Build history of the part. All positions in model axes, mm. Round coordinates to 2 decimals unless told otherwise and drop trailing zeros. Write each loop counter-clockwise with the first axis right and the second up, starting at its lowest first coordinate (ties: lowest second). Pieces come first, ordered by that corner, then holes.
Item 1: Band-saw the part on B-B, the plane z = 2.7. Count the separate pieces of the cut face and the enclosed holes in it, then the cut area to 3 significant figures.
Item 2: Drop flat-ended pins along their axis: pin 1 Ø12 at (x, y) = (-149.3, 205.49) entering from -Z; pin 2 Ø9.5 at (x, y) = (-149.3, -205.49) entering from -Z; pin 3 Ø2 at (x, z) = (-147.5, 2.5) entering from +Y; pin 4 Ø1.5 at (y, z) = (166, 3.5) entering from +X. Give the stop position or say it passes through.
Item 3: Band-saw the part on A-A, the plane y = 0. Write the cut outline in (x, z).
Item 4: Band-saw the part on C-C, the plane x = -118. Write the cut outline in (y, z), then the cut area to 3 significant figures.
Item 5: Wall check: probe 1 along Y at (x, z) = (0, 3.3); probe 2 along Y at (x, z) = (-146.5, 0.6); probe 3 along X at (y, z) = (-77, 5.5). Give the ranges that are in metal, low to high.
Item 6: Band-saw the part on D-D, the plane y = -107. Write the cut outline in (x, z).
```python
from build123d import *

# Parameters (mm, degrees)
F0_R     = 300
F0_R_2   = 5.25
F0_R_3   = 26
F1_DEPTH = 6


with BuildPart() as f1:
    # F0 (on Top) → F1 (new body)
    with BuildSketch(Plane.XY):
        Circle(F0_R)
        with Locations((-149.297454, -205.490317)):
            Circle(F0_R_2, mode=Mode.SUBTRACT)
        with Locations((-241.568355, -78.490317)):
            Circle(F0_R_2, mode=Mode.SUBTRACT)
        with Locations((0, -254)):
            Circle(F0_R_2, mode=Mode.SUBTRACT)
        with Locations((149.297454, -205.490317)):
            Circle(F0_R_2, mode=Mode.SUBTRACT)
        with Locations((241.568355, -78.490317)):
            Circle(F0_R_2, mode=Mode.SUBTRACT)
        with Locations((-241.568355, 78.490317)):
            Circle(F0_R_2, mode=Mode.SUBTRACT)
        with Locations((-149.297454, 205.490317)):
            Circle(F0_R_2, mode=Mode.SUBTRACT)
        Circle(F0_R_3, mode=Mode.SUBTRACT)
        with Locations((241.568355, 78.490317)):
            Circle(F0_R_2, mode=Mode.SUBTRACT)
        with Locations((149.297454, 205.490317)):
            Circle(F0_R_2, mode=Mode.SUBTRACT)
        with Locations((0, 254)):
            Circle(F0_R_2, mode=Mode.SUBTRACT)
    extrude(amount=F1_DEPTH)


solid = f1.part
```
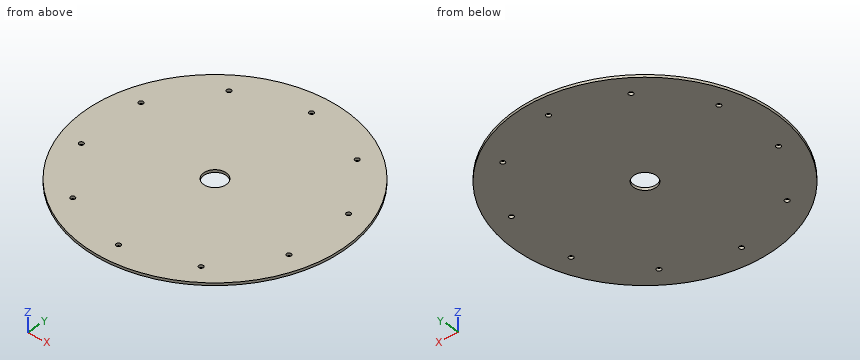
Results:
1. separate pieces: 1
1. enclosed holes: 11
1. area: 280,000 mm2
2. pin 1: stops at z = 0
2. pin 2: passes through
2. pin 3: stops at y = 261.8
2. pin 4: stops at x = 250.38
3. outline: (-300, 0) - (-26, 0) - (-26, 6) - (-300, 6) - close; (26, 0) - (300, 0) - (300, 6) - (26, 6) - close
4. outline: (-275.82, 0) - (275.82, 0) - (275.82, 6) - (-275.82, 6) - close
4. area: 3,310 mm2
5. probe 1: y = -300 to -259.25, -248.75 to -26, 26 to 248.75, 259.25 to 300
5. probe 2: y = -261.8 to -209.93, -201.05 to 201.05, 209.93 to 261.8
5. probe 3: x = -289.95 to -246.6, -236.53 to 236.53, 246.6 to 289.95
6. outline: (-280.27, 0) - (280.27, 0) - (280.27, 6) - (-280.27, 6) - close
